For this review, take the finished solid that the model builds, in its own axes (mm). Face numbers are marked on the shaded views. A direction names the side the tool comes from. Coordinates: 2 decimals unless noted, no trailing zeros. Loops run counter-clockwise (first coordinate to the right, second up) from the corner with the lowest first, then second, coordinate; pieces in that order, holes last. Notation, with made-up numbers: M 75.5,61 L 131.5,61 A31 ccw 131.5,93 Z; hole C -12,-20 d11. An arc over 180 degrees is marked long. Answer as a JSON object with one key per item and string values. Group by question number.
Item 1: Insertion check: pin 1 (1 mm diameter, centred on x = -10.5, z = 2, fed in from +Y); pin 2 (3.5 mm diameter, centred on x = -32.5, z = 7.5, fed in from +Y); pin 3 (0.9 mm diameter, centred on y = 9, z = 7, fed in from -X). Each pin has a flat end and moves straight along its axis. Give the tip position at first contact, or say it passes through.
Item 2: Mouldability with a two-part tool opening along Z and no side actions: class the marked faces 3, 4 and 5 as +Z half, -Z half, draft (parallel to the pull), parting line (faces both ways), or undercut.
Item 3: Add section C-C (y = 5). State the section outline as (x, z) points.
Item 4: Add section D-D (x = -19.5). State the section outline as (y, z) points, then the cut area to 3 significant figures.
Item 5: Wall thickness on L1, parallel to Z at x = -26.5, y = 7.25; L2, parallel to Y at x = -8.5, z = 1.75; L3, parallel to Y at x = -25, z = 7.25: over which ranges is each line inside the solid? List them lowest first. Write a range as from..to.
Item 6: Tool access review of the marked faces 1 and 2: name each direction out of +Z, -Z, +X, -X, +Y, -Y from which nothing blocks a thin tool from reaching the whole face with its end or side.
Item 7: Add section A-A (y = 8). State the section outline as (x, z) points, then the cut area to 3 significant figures.
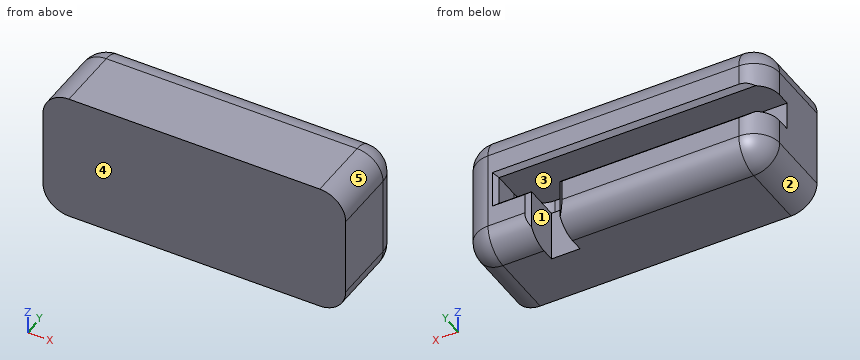
Autodesk Inventor part; units mm, degrees
ref_plane "YZ Plane" through (0, 0, 0) normal (1, 0, 0) x (0, 1, 0)
ref_plane "XZ Plane" through (0, 0, 0) normal (0, 1, 0) x (-1, 0, 0)
ref_plane "XY Plane" through (0, 0, 0) normal (0, 0, 1) x (1, 0, 0)
sketch "Sketch1" plane through (0, 0, 0) normal (0, 1, 0) x (-1, 0, 0)
  line L0 (0, 0) -> (35, 0)
  line L1 (35, 0) -> (35, 15)
  line L2 (35, 15) -> (0, 15)
  line L3 (0, 15) -> (0, 0)
  dimension "d0" = 35
  dimension "d1" = 15
extrude "Extrusion1" add sketch "Sketch1" along normal blind 4
sketch "Sketch2" plane through (0, 4, 0) normal (0, 1, 0) x (1, 0, 0)
  line L0 (0, 0) -> (-35, 0)
  line L1 (-35, 0) -> (-35, -15)
  line L2 (-35, -15) -> (0, -15)
  line L3 (0, -15) -> (0, 0)
  line L4 (-35, -5.85) -> (-31, -5.85)
  line L5 (-35, -9.15) -> (0, -9.15)
  line L6 (-17.5, -15) -> (-17.5, -9.15) construction
  line L7 (-17.5, -5.85) -> (-17.5, 0) construction
  line L8 (-31, -5.85) -> (-31, -9.15)
  line L9 (-4, -5.85) -> (-4, -9.15)
  line L10 (-4, -5.85) -> (0, -5.85)
  line L11 (-31, -5.85) -> (-4, -5.85)
  dimension "d4" = 3.3
  dimension "d7" = 27
extrude "Extrusion2" add sketch "Sketch2" along normal blind 2 contours L3 L10 L11 L4 L1 L0 | L3 L5 L9 L10 | L4 L8 L5 L1 | L3 L2 L1 L5
sketch "Sketch3" plane through (0, 6, 0) normal (0, 1, 0) x (1, 0, 0)
  line L0 (0, -15) -> (0, 0)
  line L1 (0, 0) -> (-35, 0)
  line L2 (-35, 0) -> (-35, -15)
  line L3 (-35, -15) -> (0, -15)
  line L4 (-4, -9.15) -> (-31, -9.15)
  line L5 (-31, -9.15) -> (-31, -5.85)
  line L6 (-31, -5.85) -> (-4, -5.85)
  line L7 (-4, -5.85) -> (-4, -9.15)
  line L8 (-31, -5.85) -> (-35, -5.85)
  line L9 (-31, -9.15) -> (-35, -9.15)
  line L10 (-7.75, -5.85) -> (-7.75, 0)
  line L11 (-11.05, -5.85) -> (-11.05, 0)
  line L12 (-11.05, -2.925) -> (-7.75, -2.925) construction
  dimension "d16" = 3.75
extrude "Extrusion3" add sketch "Sketch3" along normal blind 4.5 contours L3 L2 L9 L4 L7 L6 L10 L1 L0 | L11 L6 L8 L2 L1
chamfer "Chamfer3" distance 2 angle 45 1 edges at (-31, 4, 7.5)
fillet "Fillet3" radius 3 1 edges at (-4, 4, 7.5)
chamfer "Chamfer2" distance 0.5 angle 45 6 edges at (-19.5, 10.5, 9.15) (-23.025, 10.5, 5.85) (-5.875, 10.5, 5.85) (-4, 10.5, 7.5) (-7.75, 10.5, 2.925) (-11.05, 10.5, 2.925)
fillet "Fillet2" radius 3 10 edges at (0, 5.25, 15) (0, 5.25, 0) (-35, 5.25, 15) (-35, 5.25, 0) (-3.625, 10.5, 0) (0, 10.5, 7.5) (-17.5, 10.5, 15) (-23.275, 10.5, 0) (-35, 10.5, 2.675) (-35, 10.5, 12.325)
properties part number "Apoyo frontal"
From the geometry:
{
 "1": {"pin 1": "stops at y = 6", "pin 2": "stops at y = 10.1", "pin 3": "stops at x = -4"},
 "2": {"face 3": "undercut", "face 4": "draft", "face 5": "+Z half"},
 "3": {"outline": "M -35,3 A3 ccw -32,0 L -3,0 A3 ccw 0,3 L 0,12 A3 ccw -3,15 L -32,15 A3 ccw -35,12 Z; hole M -30,5.85 L -4.76,5.85 L -4.76,9.15 L -30,9.15 Z"},
 "4": {"outline": "M 0,0 L 7.5,0 A3 ccw 10.5,3 L 10.5,5.35 L 10,5.85 L 4,5.85 L 4,9.15 L 10,9.15 L 10.5,9.65 L 10.5,12 A3 ccw 7.5,15 L 0,15 Z", "area": "132 mm²"},
 "5": {"L1": "z = 0..5.85, 9.15..15", "L2": "y = 0..6", "L3": "y = 0..4"},
 "6": {"face 1": "-Z, +Y", "face 2": "-Z, -X, +Y, -Y"},
 "7": {"outline": "M -34.96,3 A2.96 ccw -32,0.04 L -11.05,0.04 L -11.05,5.85 L -34.96,5.85 Z; M -34.96,9.15 L -4,9.15 L -4,5.85 L -7.75,5.85 L -7.75,0.04 L -3,0.04 A2.96 ccw -0.04,3 L -0.04,12 A2.96 ccw -3,14.96 L -32,14.96 A2.96 ccw -34.96,12 Z", "area": "392 mm²"}
}
